```python
from build123d import *

# Parameters (mm, degrees)
SKETCH1_W           = 165.1
SKETCH1_H           = 101.6
BOSS_EXTRUDE1_DEPTH = 25
SHELL1_T            = -2
SKETCH2_W           = 5
SKETCH2_H           = 15
CUT_EXTRUDE1_DEPTH  = 25
CUT_EXTRUDE2_REACH  = 176.538
FILLET1_R           = 5
FILLET2_R           = 3
FILLET3_R           = 2
FILLET4_R           = 5
CUT_EXTRUDE3_REACH  = 176.538
SKETCH4_W           = 91.6
SKETCH4_H           = 4.4
BOSS_EXTRUDE4_START = -2.2
BOSS_EXTRUDE4_DEPTH = 2.2
BOSS_EXTRUDE2_START = 2
BOSS_EXTRUDE2_DEPTH = 2
LPATTERN1_COUNT     = 2
LPATTERN1_PITCH     = 4.2
BOSS_EXTRUDE3_DEPTH = 25
CUT_EXTRUDE4_REACH  = 182.513


with BuildPart() as part:
    # Sketch1 → Boss-Extrude1 (new body)
    with BuildSketch(Plane(origin=(0, 0, 0), x_dir=(1, 0, 0), z_dir=(0, 1, 0))):
        Rectangle(SKETCH1_W, SKETCH1_H)
    extrude(amount=BOSS_EXTRUDE1_DEPTH)

    # Shell1
    shell1_openings = [part.faces().sort_by_distance(p)[0] for p in [
        (0, 25, 0),
    ]]
    offset(amount=SHELL1_T, openings=shell1_openings, kind=Kind.INTERSECTION)

    # Sketch2 → Cut-Extrude1 (cut)
    with BuildSketch(Plane(origin=(0, 2, 0), x_dir=(1, 0, 0), z_dir=(0, 1, 0))):
        with Locations((-69.85, 37.3)):
            Rectangle(SKETCH2_W, SKETCH2_H)
    extrude(amount=-CUT_EXTRUDE1_DEPTH, mode=Mode.SUBTRACT)

    # Sketch3 → Cut-Extrude2 (cut, up to next)
    with BuildSketch(Plane(origin=(82.55, 0, 0), x_dir=(0, 0, -1), z_dir=(1, 0, 0)), mode=Mode.PRIVATE) as cut_extrude2_sk1:
        with BuildLine():
            Line((-15, 40), (15, 40))
            Line((15, 40), (15, 12))
            ThreePointArc((15, 12), (14.414213562, 10.585786438), (13, 10))
            Line((13, 10), (-13, 10))
            ThreePointArc((-13, 10), (-14.414213562, 10.585786438), (-15, 12))
            Line((-15, 12), (-15, 40))
        make_face()
    cut_extrude2_tool1 = extrude(cut_extrude2_sk1.sketch, amount=-CUT_EXTRUDE2_REACH, mode=Mode.PRIVATE) & part.part
    add(cut_extrude2_tool1.solids().sort_by_distance((82.55, 25.027814, 0))[0], mode=Mode.SUBTRACT)

    # Fillet1
    fillet1_edges = [part.edges().sort_by_distance(p)[0] for p in [
        (-82.55, 12.5, -50.8),
        (-82.55, 12.5, 50.8),
    ]]
    fillet(fillet1_edges, radius=FILLET1_R)

    # Fillet2
    fillet2_edges = [part.edges().sort_by_distance(p)[0] for p in [
        (-80.55, 13.5, -48.8),
        (-80.55, 13.5, 48.8),
        (80.55, 13.5, 48.8),
        (80.55, 13.5, -48.8),
    ]]
    fillet(fillet2_edges, radius=FILLET2_R)

    # Fillet3
    fillet3_edges = [part.edges().sort_by_distance(p)[0] for p in [
        (80.55, 2, 0),
        (-80.55, 2, 0),
        (0, 2, 48.8),
        (0, 2, -48.8),
        (-79.671320344, 2, -47.921320344),
        (-79.671320344, 2, 47.921320344),
        (79.671320344, 2, 47.921320344),
        (79.671320344, 2, -47.921320344),
    ]]
    fillet(fillet3_edges, radius=FILLET3_R)

    # Fillet4
    fillet4_edges = [part.edges().sort_by_distance(p)[0] for p in [
        (2.5, 0, -50.8),
        (2.5, 0, 50.8),
        (-82.55, 0, 0),
        (-81.085533906, 0, -49.335533906),
        (-81.085533906, 0, 49.335533906),
    ]]
    fillet(fillet4_edges, radius=FILLET4_R)

    # Sketch4 → Cut-Extrude3 (cut, up to next)
    with BuildSketch(Plane.ZY.offset(82.55), mode=Mode.PRIVATE) as cut_extrude3_sk1:
        with Locations((0, 25)):
            Rectangle(SKETCH4_W, SKETCH4_H)
    cut_extrude3_tool1 = extrude(cut_extrude3_sk1.sketch, amount=-CUT_EXTRUDE3_REACH, mode=Mode.PRIVATE) & part.part
    add(cut_extrude3_tool1.solids().sort_by_distance((-82.55, 25, 0))[0], mode=Mode.SUBTRACT)

    # Sketch8 → Boss-Extrude4 (add)
    with BuildSketch(Plane(origin=(0, 25, 0), x_dir=(1, 0, 0), z_dir=(0, 1, 0)).offset(BOSS_EXTRUDE4_START)):
        with BuildLine():
            Line((-77.55, -48.8), (77.55, -48.8))
            ThreePointArc((77.55, -48.8), (79.671320344, -47.921320344), (80.55, -45.8))
            Line((80.55, -45.8), (-80.55, -45.8))
            ThreePointArc((-80.55, -45.8), (-79.671320344, -47.921320344), (-77.55, -48.8))
        make_face()
        with BuildLine():
            Line((77.55, 48.8), (-77.55, 48.8))
            ThreePointArc((-77.55, 48.8), (-79.671320344, 47.921320344), (-80.55, 45.8))
            Line((-80.55, 45.8), (80.55, 45.8))
            ThreePointArc((80.55, 45.8), (79.671320344, 47.921320344), (77.55, 48.8))
        make_face()
    extrude(amount=BOSS_EXTRUDE4_DEPTH)

    # Sketch5 → Boss-Extrude2 (add)
    with BuildSketch(Plane(origin=(0, 25, 0), x_dir=(1, 0, 0), z_dir=(0, 1, 0)).offset(BOSS_EXTRUDE2_START)):
        with BuildLine():
            Line((-77.55, -50.8), (82.55, -50.8))
            Line((82.55, -50.8), (82.55, -42.8))
            Line((82.55, -42.8), (-82.55, -42.8))
            Line((-82.55, -42.8), (-82.55, -45.8))
            ThreePointArc((-82.55, -45.8), (-81.085533906, -49.335533906), (-77.55, -50.8))
        make_face()
        with BuildLine():
            Line((82.55, 50.8), (-77.55, 50.8))
            ThreePointArc((-77.55, 50.8), (-81.085533906, 49.335533906), (-82.55, 45.8))
            Line((-82.55, 45.8), (-82.55, 42.8))
            Line((-82.55, 42.8), (82.55, 42.8))
            Line((82.55, 42.8), (82.55, 50.8))
        make_face()
    boss_extrude2 = extrude(amount=-BOSS_EXTRUDE2_DEPTH)

    # LPattern1: Boss-Extrude2 ×2
    with Locations(*[(0, -i * LPATTERN1_PITCH, 0) for i in range(1, LPATTERN1_COUNT)]):
        add(boss_extrude2)

    # Sketch6 → Boss-Extrude3 (add)
    with BuildSketch(Plane.XZ):
        Polygon((82.55, -30.8), (84.55, -30.8), (87.55, -33.8), (90.55, -30.8), (90.55, -20.8), (87.55, -17.8), (84.55, -20.8), (82.55, -20.8), align=None)
        Polygon((82.55, 20.8), (82.55, 30.8), (84.55, 30.8), (87.55, 33.8), (90.55, 30.8), (90.55, 20.8), (87.55, 17.8), (84.55, 20.8), align=None)
    extrude(amount=-BOSS_EXTRUDE3_DEPTH)

    # Sketch7 → Cut-Extrude4 (cut, up to next)
    with BuildSketch(Plane(origin=(-80.55, 0, 0), x_dir=(0, 0, -1), z_dir=(1, 0, 0)), mode=Mode.PRIVATE) as cut_extrude4_sk1:
        with BuildLine():
            Line((11.519977141, 20.8), (-9.480022859, 20.8))
            ThreePointArc((-9.480022859, 20.8), (-10.894236421, 20.214213562), (-11.480022859, 18.8))
            Line((-11.480022859, 18.8), (-11.480022859, 7.8))
            ThreePointArc((-11.480022859, 7.8), (-10.894236421, 6.385786438), (-9.480022859, 5.8))
            Line((-9.480022859, 5.8), (11.519977141, 5.8))
            ThreePointArc((11.519977141, 5.8), (12.934190704, 6.385786438), (13.519977141, 7.8))
            Line((13.519977141, 7.8), (13.519977141, 18.8))
            ThreePointArc((13.519977141, 18.8), (12.934190704, 20.214213562), (11.519977141, 20.8))
        make_face()
    cut_extrude4_tool1 = extrude(cut_extrude4_sk1.sketch, amount=-CUT_EXTRUDE4_REACH, mode=Mode.PRIVATE) & part.part
    add(cut_extrude4_tool1.solids().sort_by_distance((-80.55, 13.3, -1.019977))[0], mode=Mode.SUBTRACT)


solid = part.part
```
The listing builds one solid part. Answer for the finished solid, in the listing's coordinates (mm). A direction names the side the tool comes from. Coordinates: 2 decimals unless noted, no trailing zeros. Write each loop counter-clockwise with the first axis right and the second up, starting at its lowest first coordinate (ties: lowest second). Pieces come first, ordered by that corner, then holes. Notation, with made-up numbers: (53.25, 37) - (101.25, 37) arc R33 ccw to (101.25, 70) - close; hole circle Ø10 at (71, -5). An arc over 180 degrees is marked (long way). One line per item, written item: value.
1) Find section D-D (z = 3). Give the vertices of the cut face in (x, y).
Geometry check:
outline: (-82.55, 5) arc R5 ccw to (-77.55, 0) - (82.55, 0) - (82.55, 10) - (80.55, 10) - (80.55, 4) arc R2 cw to (78.55, 2) - (-78.55, 2) arc R2 cw to (-80.55, 4) - (-80.55, 5.8) - (-82.55, 5.8) - close; (-82.55, 20.8) - (-80.55, 20.8) - (-80.55, 22.8) - (-82.55, 22.8) - close
2) Each of these flat-tipped pins is pushed along its axis until it touches: pin 1 Ø3 at (x, y) = (23.5, 4) entering from +Z; pin 2 Ø10 at (y, z) = (8.5, -42) entering from +X; pin 3 Ø8 at (x, z) = (52, 20) entering from +Y; pin 4 Ø0.6 at (x, z) = (-82, -2.5) entering from +Y. Where does it stop, or does it pass through?
Geometry check:
pin 1: stops at z = 50.8
pin 2: stops at x = 82.55
pin 3: stops at y = 2
pin 4: stops at y = 22.8
3) Find section A-A (z = -39.5). Give the vertices of the cut face in (x, y).
Geometry check:
outline: (-82.55, 5) arc R5 ccw to (-77.55, 0) - (-72.35, 0) - (-72.35, 2) - (-78.55, 2) arc R2 cw to (-80.55, 4) - (-80.55, 22.8) - (-82.55, 22.8) - close; (-67.35, 0) - (82.55, 0) - (82.55, 25) - (80.55, 25) - (80.55, 4) arc R2 cw to (78.55, 2) - (-67.35, 2) - close
4) A tool of negligible diameter and unlimited length cuts with its end or side. For faces 5 (the flat face through (-1, 22.8, -44)), 6 (the flat face through (-1, 27, -47)), 7 (the flat face through (-1, 20.8, 46)), from which of +Z, -Z, +X, -X, +Y, -Y can it reach the whole face along a straight path? Write none if from no direction.
Geometry check:
face 5: -X
face 6: +Z, -Z, +X, -X, +Y
face 7: none
5) Find section B-B (x = 42.5). Give the vertices of the cut face in (y, z).
Geometry check:
outline: (0, -45.8) arc R5 ccw to (5, -50.8) - (27, -50.8) - (27, -42.8) - (25, -42.8) - (25, -45.8) - (22.8, -45.8) - (22.8, -42.8) - (20.8, -42.8) - (20.8, -48.8) - (4, -48.8) arc R2 cw to (2, -46.8) - (2, 46.8) arc R2 cw to (4, 48.8) - (20.8, 48.8) - (20.8, 42.8) - (22.8, 42.8) - (22.8, 45.8) - (25, 45.8) - (25, 42.8) - (27, 42.8) - (27, 50.8) - (5, 50.8) arc R5 ccw to (0, 45.8) - close
6) Find section C-C (z = 29). Give the vertices of the cut face in (x, y).
Geometry check:
outline: (-82.55, 5) arc R5 ccw to (-77.55, 0) - (90.55, 0) - (90.55, 25) - (80.55, 25) - (80.55, 4) arc R2 cw to (78.55, 2) - (-78.55, 2) arc R2 cw to (-80.55, 4) - (-80.55, 22.8) - (-82.55, 22.8) - close
7) Consider line 1 along Y through (x, z) = (67.5, 43); line 2 along X through (y, z) = (20.25, 23); line 3 along Z through (x, y) = (13.5, 24). Determine where each line is inside the solid, lowest interval first. Write a range as from..to.
Geometry check:
line 1: y = 0..2, 20.8..22.8, 25..27
line 2: x = -82.55..-80.55, 80.55..90.55
line 3: z = -50.8..-45.8, 45.8..50.8
8) For a pull along Z with two mould halves and no side action, classify faces 1 (the flat face through (82.55, 7, 0)), 2 (the flat face through (-80.55, 5, 1)), 3 (the flat face through (-1, 27, 47)), 4 (the cylindrical face through (3.62, 1.5, -49.37)) as pulls with the +Z half, pulls with the -Z half, needs draft (parallel to the pull), parting line crosses it, or undercut.
Geometry check:
face 1: undercut
face 2: undercut
face 3: needs draft
face 4: pulls with the -Z half
